Could you check a few things on this model? Use its own coordinates, in mm. Face numbers are marked on the shaded views. A direction names the side the tool comes from. Give positions to 0.01 mm unless a question says otherwise; leave off trailing zeros. Write each loop counter-clockwise with the first axis right and the second up, starting at its lowest first coordinate (ties: lowest second). Pieces come first, ordered by that corner, then holes. Notation, with made-up numbers: M 0,-32 L 24,-32 A22 ccw 24,-8 Z; hole C 31,15.5 d5. An arc over 180 degrees is marked long. Use one line per item in the form item = value.
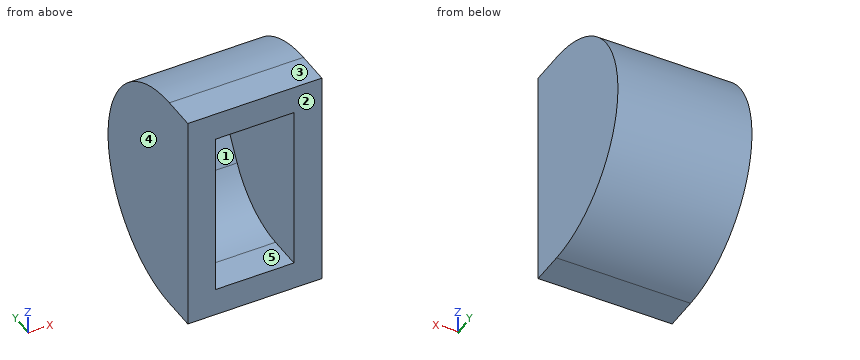
from build123d import *

# Parameters (mm, degrees)
BOSS_EXTRUDE1_DEPTH = 6
CUT_EXTRUDE1_DEPTH  = 3.5


with BuildPart() as part:
    # Sketch1 → Boss-Extrude1 (new body, symmetric)
    with BuildSketch(Plane(origin=(0, 0, 0), x_dir=(0, 0, -1), z_dir=(1, 0, 0))):
        with BuildLine():
            Line((0, 0), (0, 3))
            ThreePointArc((0, 3), (10, 13), (20, 3))
            Line((20, 3), (20, 0))
            Line((20, 0), (0, 0))
        make_face()
    extrude(amount=BOSS_EXTRUDE1_DEPTH, both=True)

    # Sketch2 → Cut-Extrude1 (cut, symmetric)
    with BuildSketch(Plane(origin=(0, 0, 0), x_dir=(0, 0, -1), z_dir=(1, 0, 0))):
        with BuildLine():
            Line((10, 0), (17.5, 0))
            Line((17.5, 0), (17.5, 3))
            ThreePointArc((17.5, 3), (16.532377607, 6.611215932), (13.888784068, 9.254809472))
            Line((13.888784068, 9.254809472), (10, 11.5))
            Line((10, 11.5), (6.111215932, 9.254809472))
            ThreePointArc((6.111215932, 9.254809472), (3.467622393, 6.611215932), (2.5, 3))
            Line((2.5, 3), (2.5, 0))
            Line((2.5, 0), (10, 0))
        make_face()
    extrude(amount=CUT_EXTRUDE1_DEPTH, both=True, mode=Mode.SUBTRACT)


solid = part.part
1) Thinking about a two-plate mould opening in X: for the marked faces 3, 4 and 5, which applies, released by +X, released by -X, zero draft, split by the parting line, or undercut?
Checked values:
face_3 = zero draft
face_4 = released by -X
face_5 = undercut
2) I want a section at A-A, the plane y = 2.75. Please give me the cut outline in (x, z).
Checked values:
outline = M -6,-20 L 6,-20 L 6,0 L -6,0 Z; hole M -3.5,-17.5 L 3.5,-17.5 L 3.5,-2.5 L -3.5,-2.5 Z
3) For the marked faces 1 and 2, which set-ups out of +Z, -Z, +X, -X, +Y, -Y let a thin tool reach every point of the face, with its end or its side?
Checked values:
face_1 = -Y
face_2 = +Z, -Z, +X, -X, -Y
4) For pin 1 Ø2 at (x, y) = (-2.5, 11.5) entering from -Z; pin 2 Ø1.5 at (x, z) = (-1, -10.5) entering from -Y; pin 3 Ø3 at (x, y) = (1, 9) entering from +Z, each with a flat end and sliding along its axis, tell me the tip position at first contact or that it passes through.
Checked values:
pin_1 = -16.61
pin_2 = 10.78
pin_3 = -1.07
5) I want a section at D-D, the plane y = 6.5. Please give me the cut outline in (x, z).
Checked values:
outline = M -6,-19.37 L 6,-19.37 L 6,-0.63 L -6,-0.63 Z; hole M -3.5,-16.6 L 3.5,-16.6 L 3.5,-3.4 L -3.5,-3.4 Z
6) I want a section at C-C, the plane z = -13. Please give me the cut outline in (x, y), plus the area to 3 significant figures.
Checked values:
outline = M -6,0 L -3.5,0 L -3.5,9.77 L 3.5,9.77 L 3.5,0 L 6,0 L 6,12.54 L -6,12.54 Z
area = 82.1 mm2
7) If I drill on L1, parallel to X at y = 2.5, z = -8; L2, parallel to Z at x = 1, y = 1.5; L3, parallel to Z at x = 3.25, y = 5.75, over which ranges is the centre line in solid material (lowest first)?
Checked values:
L1 = -6 to -3.5, 3.5 to 6
L2 = -20 to -17.5, -2.5 to 0
L3 = -19.61 to -16.96, -3.04 to -0.39
8) I want a section at B-B, the plane x = -2.5. Please give me the cut outline in (y, z).
Checked values:
outline = M 0,-20 L 3,-20 A10 ccw 3,0 L 0,0 L 0,-2.5 L 3,-2.5 A7.22 cw 9.25,-6.11 L 11.5,-10 L 9.25,-13.89 A7.22 cw 3,-17.5 L 0,-17.5 Z
